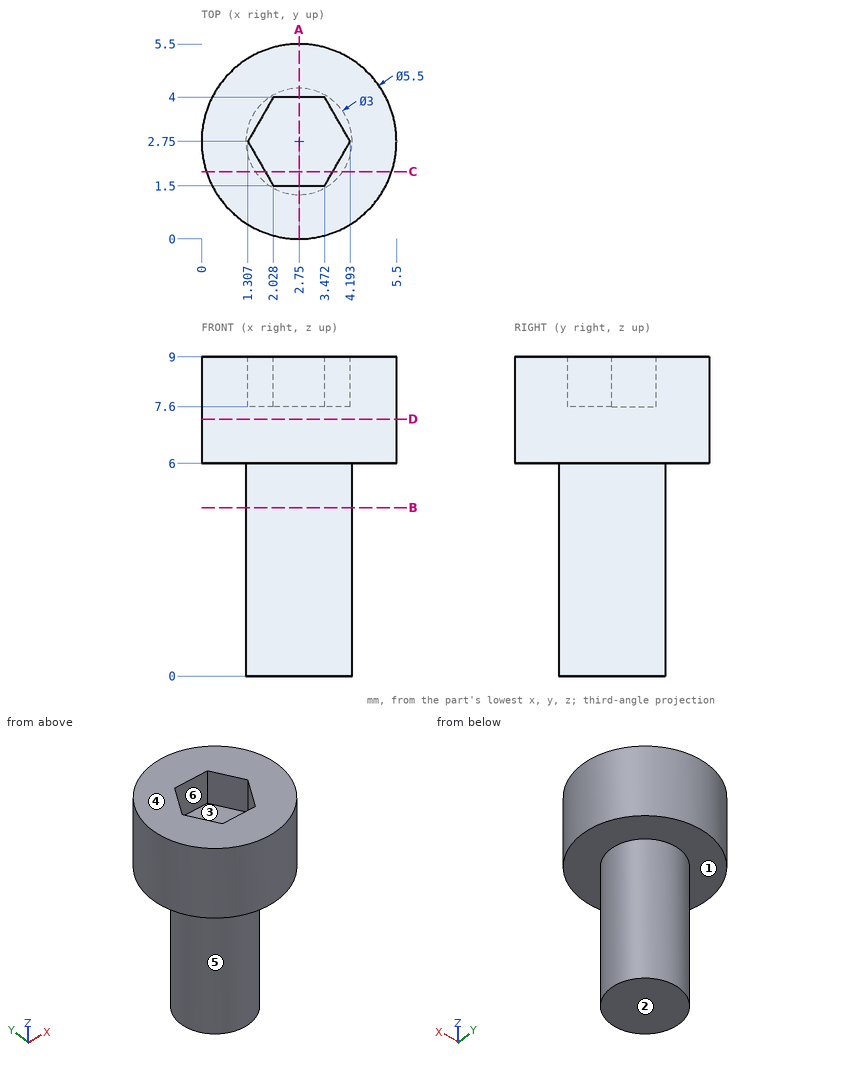
Check sheet for the drawn part. Datum: minimum x, y, z corner. Units: mm. A direction names the side the tool comes from. Round coordinates to 2 decimals unless told otherwise and drop trailing zeros. Write each loop counter-clockwise with the first axis right and the second up, starting at its lowest first coordinate (ties: lowest second). Pieces come first, ordered by that corner, then holes. Notation, with made-up numbers: (-8, 88) - (49, 88) arc R32 ccw to (49, 126) - close; hole circle Ø8 at (81, 22). An arc over 180 degrees is marked (long way). Write each question's results on one line, items separated by ' | '.
(1) Sectioned sample at A-A, the plane x = 2.75. Enter the section's corners in (y, z).
Computed:
outline: (0, 6) - (1.25, 6) - (1.25, 0) - (4.25, 0) - (4.25, 6) - (5.5, 6) - (5.5, 9) - (4, 9) - (4, 7.6) - (1.5, 7.6) - (1.5, 9) - (0, 9) - close
(2) Sectioned sample at C-C, the plane y = 1.9. Enter the section's corners in (x, z) (1 decimal).
Computed:
outline: (0.1, 6) - (1.5, 6) - (1.5, 0) - (4, 0) - (4, 6) - (5.4, 6) - (5.4, 9) - (3.7, 9) - (3.7, 7.6) - (1.8, 7.6) - (1.8, 9) - (0.1, 9) - close
(3) Sectioned sample at B-B, the plane z = 4.75. Enter the section's corners in (x, y).
Computed:
outline: circle Ø3 at (2.75, 2.75)
(4) Set-up check for the marked faces 1, 2 and 3: record each of +Z, -Z, +X, -X, +Y, -Y from which the full face is reachable in a straight line by a thin tool's end or side.
Computed:
face 1: -Z | face 2: -Z, +X, -X, +Y, -Y | face 3: +Z
(5) Depth check by flat-ended pin: pin 1 Ø3 at (x, z) = (1, 1.5) entering from +Y. Enter the tip coordinate at first touch or a pass-through.
Computed:
pin 1: stops at y = 4.23
(6) Draft check along Y on the marked faces 4, 5 and 6. Enter one of: pulls with the +Y half, pulls with the -Y half, needs draft (parallel to the pull), parting line crosses it, or undercut.
Computed:
face 4: needs draft | face 5: parting line crosses it | face 6: undercut
(7) Thickness scan on probe 1 along Z at (x, y) = (4.4, 4.8); probe 2 along Y at (x, z) = (1.9, 8.75) (1 decimal); probe 3 along X at (y, z) = (1.9, 8.75) (1 decimal). Record the ranges inside material, lowest first. Write a range as from..to.
Computed:
probe 1: z = 6..9 | probe 2: y = 0.1..1.7, 3.8..5.4 | probe 3: x = 0.1..1.8, 3.7..5.4
(8) Sectioned sample at D-D, the plane z = 7.25. Enter the section's corners in (x, y).
Computed:
outline: circle Ø5.5 at (2.75, 2.75)
